The drawing under review shows one solid part. Ordinate dimensions are in mm from its lowest x, y, z. A direction names the side the tool comes from. Give positions to 0.01 mm unless a question says otherwise; leave off trailing zeros. Order: outer loops, then holes, each group sorted by start corner. A loop starts at its lowest first (then second) coordinate and runs counter-clockwise, first axis right, second up. Notation, with made-up numbers: (3.5, 4) -> (41.5, 4) arc R22 cw to (41.5, 22) -> close; hole circle Ø9 at (60, -6.5). An arc over 180 degrees is marked (long way). Return JSON: item names as keys, results as strings. Group by question number.
1) For the marked faces 1 and 2, list the 3-axis set-ups (+Z, -Z, +X, -X, +Y, -Y) from which the entire face can be reached by the end or side of a thin tool; tool diameter is ignored.
2) Add section A-A (x = 7.5). Give the boundary of the cut face in (y, z), then the cut area to 3 significant figures.
3) To check wall thickness, follow line 1 along Z through (x, y) = (7.5, 0.8); line 2 along X through (y, z) = (1.25, 5); line 3 along Y through (x, z) = (6, 24.75). State the ranges of each line that lie inside material, in increasing order.
4) Insertion check: P1, Ø2, axis at x = 7, y = 5.5, coming from the -Z side; P2, Ø7, axis at x = 10.5, z = 19.5, coming from the -Y side; P3, Ø8, axis at x = 1.5, z = 7.5, coming from the +Y side; P4, Ø5, axis at x = 7, z = 4.5, coming from the +Y side. Each pin has a flat end and moves straight along its axis. Give the tip position at first contact, or say it passes through.
5) The part is to be moulded in two halves that separate along Z. For the marked faces 3, 4 and 5, say which applies: released by +Z, released by -Z, zero draft, split by the parting line, or undercut.
6) Add section B-B (z = 5). Give the boundary of the cut face in (x, y).
7) Add section D-D (y = 9.75). Give the boundary of the cut face in (x, z).
8) Add section C-C (x = 2). Give the boundary of the cut face in (y, z).
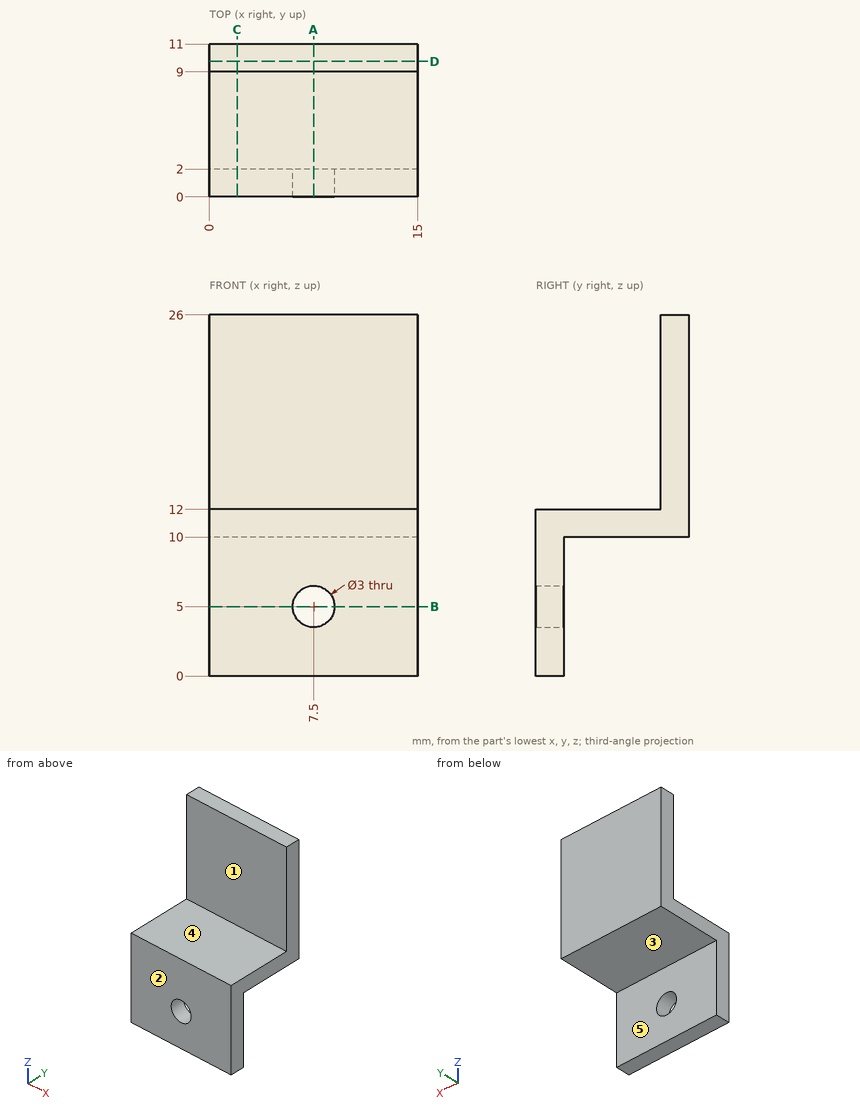
Evaluation:
{
 "1": {"face 1": "+Z, +X, -X, -Y", "face 2": "+Z, -Z, +X, -X, -Y"},
 "2": {"outline": "(0, 0) -> (2, 0) -> (2, 3.5) -> (0, 3.5) -> close; (0, 6.5) -> (2, 6.5) -> (2, 10) -> (11, 10) -> (11, 26) -> (9, 26) -> (9, 12) -> (0, 12) -> close", "area": "64.0 mm^2"},
 "3": {"line 1": "0 to 3.5, 6.5 to 12", "line 2": "0 to 6, 9 to 15", "line 3": "9 to 11"},
 "4": {"P1": "z = 10", "P2": "y = 9", "P3": "y = 11", "P4": "y = 2"},
 "5": {"face 3": "released by -Z", "face 4": "released by +Z", "face 5": "zero draft"},
 "6": {"outline": "(0, 0) -> (6, 0) -> (6, 2) -> (0, 2) -> close; (9, 0) -> (15, 0) -> (15, 2) -> (9, 2) -> close"},
 "7": {"outline": "(0, 10) -> (15, 10) -> (15, 26) -> (0, 26) -> close"},
 "8": {"outline": "(0, 0) -> (2, 0) -> (2, 10) -> (11, 10) -> (11, 26) -> (9, 26) -> (9, 12) -> (0, 12) -> close"}
}
